Can you work these out from the model? Positions are in its coordinate system, mm. Face numbers are marked on the shaded views. Give positions to 0.01 mm unless a question says otherwise; leave off trailing zeros. Loops run counter-clockwise (first coordinate to the right, second up) from the corner with the lowest first, then second, coordinate; pieces in that order, holes last. Notation, with made-up numbers: (-27.5, -21) - (18.5, -21) arc R16 cw to (18.5, 8) - close; hole circle Ø10 at (61, -22.5). An arc over 180 degrees is marked (long way). Answer as a JSON object with one key per item and string values. Group by question number.
Item 1: Thinking about a two-plate mould opening in Z: for the marked faces 1 and 2, which applies, pulls with the +Z half, pulls with the -Z half, needs draft (parallel to the pull), parting line crosses it, or undercut?
Item 2: Suppose I cut it at A-A on y = 10.85. Write out the boundary of the cut face in (x, z), and give its area (3 significant figures).
Item 3: Suppose I cut it at B-B on x = -11. Write out the boundary of the cut face in (y, z).
Item 4: Please list where these lines run through material, in increasing order: L1, parallel to Z at x = -13, y = 12.5; L2, parallel to Y at x = -3.5, z = -21.
Item 5: Will this pin go through, and if not, where does the flat tip stop? pin 1 (1 mm diameter, centred on x = -63, y = 12.5, fed in from +Z).
Item 6: Suppose I cut it at C-C on z = -23. Write out the boundary of the cut face in (x, y).
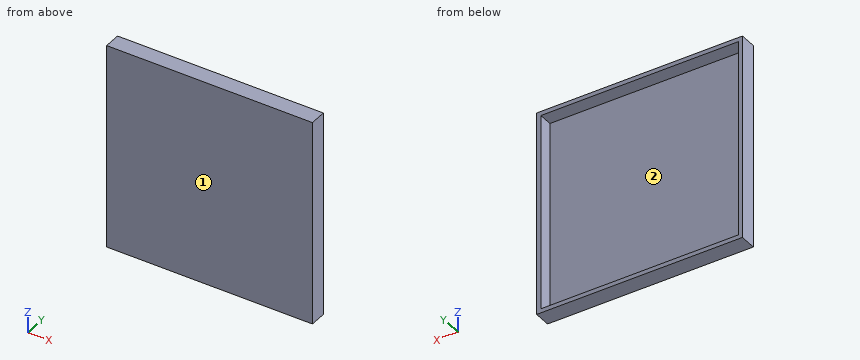
Autodesk Inventor part; units mm, degrees
ref_plane "YZ Plane" through (0, 0, 0) normal (1, 0, 0) x (0, 1, 0)
ref_plane "XZ Plane" through (0, 0, 0) normal (0, 1, 0) x (-1, 0, 0)
ref_plane "XY Plane" through (0, 0, 0) normal (0, 0, 1) x (1, 0, 0)
sketch "Sketch1" plane through (0, 0, 0) normal (0, 1, 0) x (-1, 0, 0)
  line L0 (0, 0) -> (74, 0)
  line L1 (74, 0) -> (74, -74)
  line L2 (74, -74) -> (0, -74)
  line L3 (0, -74) -> (0, 0)
  dimension "d0" = 74
  dimension "d1" = 74
extrude "Extrusion1" add sketch "Sketch1" along normal blind 10
sketch "Sketch2" plane through (0, 10, 0) normal (0, 1, 0) x (1, 0, 0)
  line L0 (0, 0) -> (0, 74)
  line L1 (0, 74) -> (-74, 74)
  line L2 (0, 0) -> (-74, 0)
  line L3 (-74, 0) -> (-74, 74)
  line L4 (-74, 74) -> (0, 74)
  line L5 (0, 74) -> (0, 0)
  line L6 (-72.5, 72.5) -> (-72.5, 1.5)
  line L7 (-72.5, 1.5) -> (-1.5, 1.5)
  line L8 (-1.5, 1.5) -> (-1.5, 72.5)
  line L9 (-1.5, 72.5) -> (-72.5, 72.5)
  dimension "d4" = 1.5
extrude "Extrusion2" add sketch "Sketch2" along normal blind 5
sketch "Sketch3" plane through (0, 0, 0) normal (0, -1, 0) x (1, 0, 0)
  line L0 (0, 0) -> (0, -74)
  line L1 (0, 0) -> (-74, 0)
  line L2 (-74, 0) -> (-74, -74)
  line L3 (-74, -74) -> (0, -74)
  line L4 (0, -74) -> (0, 0)
extrude "Extrusion3" cut sketch "Sketch3" against normal blind 5
sketch "Sketch4" plane through (0, 5, 0) normal (0, -1, 0) x (1, 0, 0)
  line L0 (0, -74) -> (-74, -74)
  line L1 (-74, 0) -> (0, 0)
  line L2 (-74, -74) -> (0, -74)
  line L3 (0, -74) -> (0, 0)
  line L4 (0, 0) -> (-74, 0)
  line L5 (-74, 0) -> (-74, -74)
extrude "Extrusion4" cut sketch "Sketch4" against normal blind 4
properties part number "DiffusorCapUltrathin"
Worked out:
{
 "1": {"face 1": "needs draft", "face 2": "undercut"},
 "2": {"outline": "(-74, -74) - (0, -74) - (0, 0) - (-74, 0) - close; hole (-72.5, -72.5) - (-1.5, -72.5) - (-1.5, -1.5) - (-72.5, -1.5) - close", "area": "435 mm2"},
 "3": {"outline": "(9, -74) - (15, -74) - (15, -72.5) - (10, -72.5) - (10, -1.5) - (15, -1.5) - (15, 0) - (9, 0) - close"},
 "4": {"L1": "z = -74 to -72.5, -1.5 to 0", "L2": "y = 9 to 10"},
 "5": {"pin 1": "stops at z = 0"},
 "6": {"outline": "(-74, 9) - (0, 9) - (0, 15) - (-1.5, 15) - (-1.5, 10) - (-72.5, 10) - (-72.5, 15) - (-74, 15) - close"}
}
